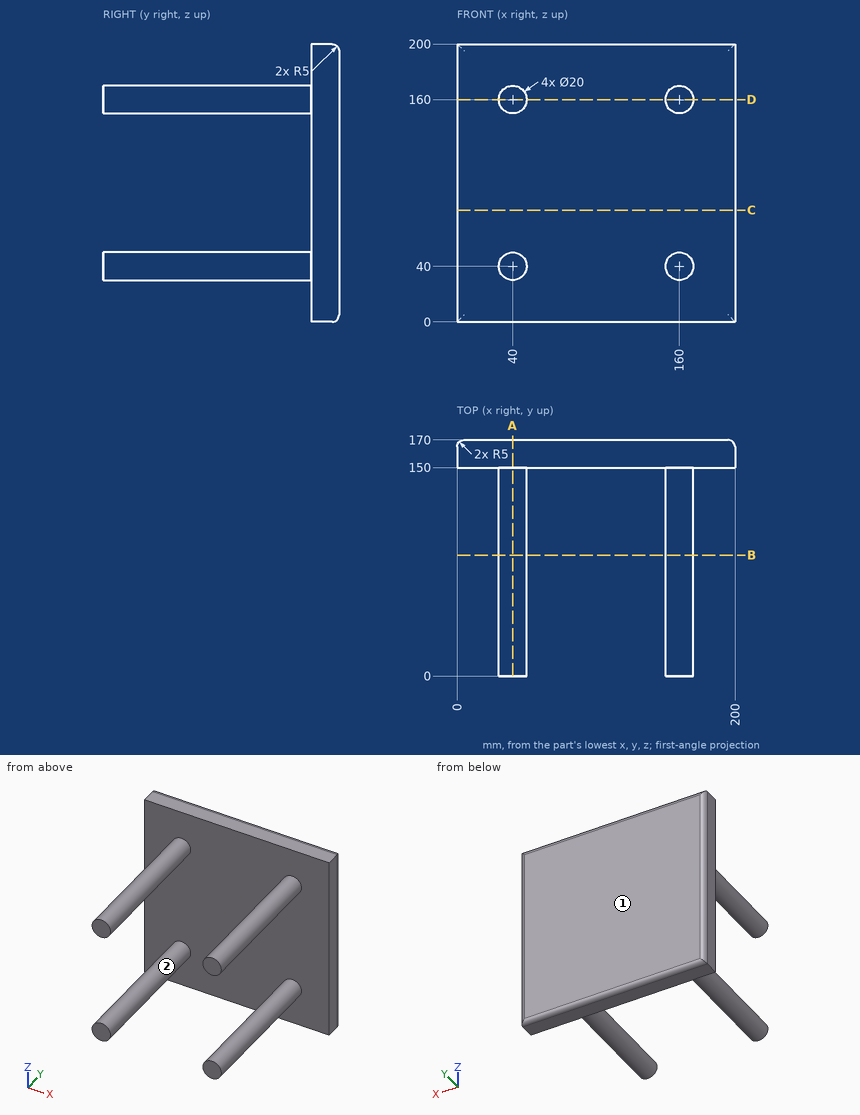
The drawing under review shows one solid part. Ordinate dimensions are in mm from its lowest x, y, z. Round coordinates to 2 decimals unless told otherwise and drop trailing zeros. Order: outer loops, then holes, each group sorted by start corner. A loop starts at its lowest first (then second) coordinate and runs counter-clockwise, first axis right, second up. Notation, with made-up numbers: (42, 51.25) -> (62, 51.25) arc R26 ccw to (62, 87.25) -> close; hole circle Ø6 at (0.5, 60.5). An arc over 180 degrees is marked (long way). Use a Markdown table: item, result.
Q1. Mouldability with a two-part tool opening along Z and no side actions: class the marked faces 1 and 2 as +Z half, -Z half, draft (parallel to the pull), parting line (faces both ways), or undercut.
Values:
| item | result |
|---|---|
| face 1 | draft |
| face 2 | undercut |
Q2. For line 1 (Y direction, x = 76.5, z = 151.5); line 2 (Z direction, x = 47.5, y = 21); line 3 (Z direction, x = 44, y = 50), list the stretches that pass through material, from the lowest coordinate up.
Values:
| item | result |
|---|---|
| line 1 | y = 150 to 170 |
| line 2 | z = 33.39 to 46.61, 153.39 to 166.61 |
| line 3 | z = 30.83 to 49.17, 150.83 to 169.17 |
Q3. We need section A-A on x = 40. Write out the cut boundary in (y, z).
Values:
| item | result |
|---|---|
| outline | (0, 30) -> (150, 30) -> (150, 0) -> (165, 0) arc R5 ccw to (170, 5) -> (170, 195) arc R5 ccw to (165, 200) -> (150, 200) -> (150, 170) -> (0, 170) -> (0, 150) -> (150, 150) -> (150, 50) -> (0, 50) -> close |
Q4. We need section B-B on y = 87. Write out the cut boundary in (x, z).
Values:
| item | result |
|---|---|
| outline | circle Ø20 at (40, 40); circle Ø20 at (40, 160); circle Ø20 at (160, 40); circle Ø20 at (160, 160) |
Q5. We need section C-C on z = 80.5. Write out the cut boundary in (x, y).
Values:
| item | result |
|---|---|
| outline | (0, 150) -> (200, 150) -> (200, 165) arc R5 ccw to (195, 170) -> (5, 170) arc R5 ccw to (0, 165) -> close |
Q6. We need section D-D on z = 160. Write out the cut boundary in (x, y).
Values:
| item | result |
|---|---|
| outline | (0, 150) -> (30, 150) -> (30, 0) -> (50, 0) -> (50, 150) -> (150, 150) -> (150, 0) -> (170, 0) -> (170, 150) -> (200, 150) -> (200, 165) arc R5 ccw to (195, 170) -> (5, 170) arc R5 ccw to (0, 165) -> close |
Q7. Clearance check with flat-ended pins moving along their axes: P1, Ø1, axis at x = 171, z = 176.5, coming from the -Y side; P2, Ø12, axis at y = 41.5, z = 145, coming from the +X side. State where each tip first meets the part, or that it passes through.
Values:
| item | result |
|---|---|
| P1 | stops at y = 150 |
| P2 | stops at x = 164.36 |
